from build123d import *

# Parameters (mm, degrees)
SKETCH2_R          = 40
CUT_EXTRUDE1_DEPTH = 10


with BuildPart() as part:
    # Sketch1 → Revolve1 (revolve)
    with BuildSketch(Plane.XY, mode=Mode.PRIVATE) as revolve1_sk:
        Polygon((0, 0), (0, 50), (2, 50), (3, 47), (7, 47), (8, 50), (10, 50), (10, 0), align=None)
    revolve(revolve1_sk.sketch.rotate(Axis((10, 0, 0), (-1, 0, 0)), 90), axis=Axis((10, 0, 0), (-1, 0, 0)))

    # Sketch2 → Cut-Extrude1 (cut)
    with BuildSketch(Plane(origin=(10, 0, 0), x_dir=(0, 0, -1), z_dir=(1, 0, 0))):
        Circle(SKETCH2_R)
    extrude(amount=-CUT_EXTRUDE1_DEPTH, mode=Mode.SUBTRACT)


solid = part.part
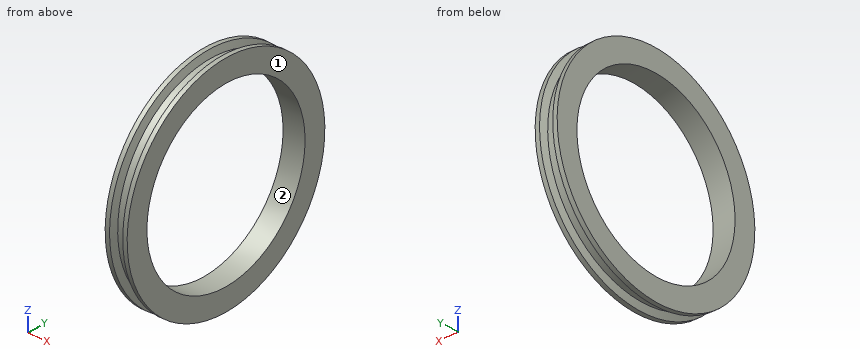
For this review, take the finished solid that the model builds, in its own axes (mm). Face numbers are marked on the shaded views. Give positions to 0.01 mm unless a question says otherwise; leave off trailing zeros. Loops run counter-clockwise (first coordinate to the right, second up) from the corner with the lowest first, then second, coordinate; pieces in that order, holes last. Notation, with made-up numbers: M 65.25,-11 L 92.25,-11 A21 ccw 92.25,9 Z; hole C 6.5,80 d10. An arc over 180 degrees is marked long. Put each result on its own line as item: value. Start each with the question number.
(1) The part is to be moulded in two halves that separate along Z. For the marked faces 1 and 2, say which applies: +Z half, -Z half, draft (parallel to the pull), parting line (faces both ways), or undercut.
(2) For pin 1 (3 mm diameter, centred on x = 5, y = 11.5, fed in from +Z), flat-tipped, find the tip position at first contact; note if it passes through.
(3) Add section A-A, the plane y = 0. Write out the cut boundary in (x, z), then the cut area to 3 significant figures.
(4) Add section C-C, the plane x = 4.25. Write out the cut boundary in (y, z), then the cut area to 3 significant figures.
(5) Wall thickness on L1, parallel to Y at x = 6, z = 0; L2, parallel to Z at x = 6, y = -19.5; L3, parallel to Y at x = 5.75, z = 7: over which ranges is each line inside the solid? List them lowest first.
Result:
1. face 1: draft
1. face 2: undercut
2. pin 1: stops at z = 45.92
3. outline: M 0,-50 L 2,-50 L 3,-47 L 7,-47 L 8,-50 L 10,-50 L 10,-40 L 0,-40 Z; M 0,40 L 10,40 L 10,50 L 8,50 L 7,47 L 3,47 L 2,50 L 0,50 Z
3. area: 170 mm^2
4. outline: C 0,0 d94; hole C 0,0 d80
4. area: 1,910 mm^2
5. L1: y = -47 to -40, 40 to 47
5. L2: z = -42.76 to -34.92, 34.92 to 42.76
5. L3: y = -46.48 to -39.38, 39.38 to 46.48
